```python
from build123d import *

# Parameters (mm, degrees)
F1_DEPTH = 7.62
F2_R     = 2.365375
F3_DEPTH = 25.4


with BuildPart() as f1:
    # F0 (on Front) → F1 (new body)
    with BuildSketch(Plane.XZ):
        Polygon((10.0597376004, 17.4239766347), (-10.0597376004, 17.4239766347), (-20.1194752008, 0), (-10.0597376004, -17.4239766347), (10.0597376004, -17.4239766347), (20.1194752008, 0), align=None)
        with BuildLine():
            add(Edge.make_bspline(
                [(-8.8631942381, -0.7304763376), (-8.451958628, -1.1782662241), (-8.451958628, -1.8910746148)],
                knots=[0, 0, 0, 1, 1, 1], degree=2))
            add(Edge.make_bspline(
                [(-8.451958628, -1.8910746148), (-8.451958628, -2.8095008106), (-9.1183126258, -3.3243068706)],
                knots=[0, 0, 0, 1, 1, 1], degree=2))
            add(Edge.make_bspline(
                [(-9.1183126258, -3.3243068706), (-9.7846666235, -3.8391129306), (-10.9269877626, -3.8391129306)],
                knots=[0, 0, 0, 1, 1, 1], degree=2))
            add(Edge.make_bspline(
                [(-10.9269877626, -3.8391129306), (-12.1637407824, -3.8391129306), (-12.8308563276, -3.5192630116)],
                knots=[0, 0, 0, 1, 1, 1], degree=2))
            Line((-12.8308563276, -3.5192630116), (-12.8308563276, -2.7394384474))
            add(Edge.make_bspline(
                [(-12.8308563276, -2.7394384474), (-12.4013435793, -2.9191636399), (-11.8971991833, -3.0242571847)],
                knots=[0, 0, 0, 1, 1, 1], degree=2))
            add(Edge.make_bspline(
                [(-11.8971991833, -3.0242571847), (-11.3930547873, -3.1293507295), (-10.8980489604, -3.1293507295)],
                knots=[0, 0, 0, 1, 1, 1], degree=2))
            add(Edge.make_bspline(
                [(-10.8980489604, -3.1293507295), (-10.0892855939, -3.1293507295), (-9.6795730788, -2.8224471168)],
                knots=[0, 0, 0, 1, 1, 1], degree=2))
            add(Edge.make_bspline(
                [(-9.6795730788, -2.8224471168), (-9.2698605636, -2.5155435042), (-9.2698605636, -1.9672293574)],
                knots=[0, 0, 0, 1, 1, 1], degree=2))
            add(Edge.make_bspline(
                [(-9.2698605636, -1.9672293574), (-9.2698605636, -1.6062558775), (-9.4153161219, -1.3755070074)],
                knots=[0, 0, 0, 1, 1, 1], degree=2))
            add(Edge.make_bspline(
                [(-9.4153161219, -1.3755070074), (-9.5607716803, -1.1447581373), (-9.9011833797, -0.9490404489)],
                knots=[0, 0, 0, 1, 1, 1], degree=2))
            add(Edge.make_bspline(
                [(-9.9011833797, -0.9490404489), (-10.2415950792, -0.7533227604), (-10.9361263317, -0.5065813943)],
                knots=[0, 0, 0, 1, 1, 1], degree=2))
            add(Edge.make_bspline(
                [(-10.9361263317, -0.5065813943), (-11.9063377524, -0.1593157681), (-12.3229041944, 0.3166513732)],
                knots=[0, 0, 0, 1, 1, 1], degree=2))
            add(Edge.make_bspline(
                [(-12.3229041944, 0.3166513732), (-12.7394706365, 0.7926185144), (-12.7394706365, 1.558735225)],
                knots=[0, 0, 0, 1, 1, 1], degree=2))
            add(Edge.make_bspline(
                [(-12.7394706365, 1.558735225), (-12.7394706365, 2.3629293069), (-12.1355635276, 2.8388964481)],
                knots=[0, 0, 0, 1, 1, 1], degree=2))
            add(Edge.make_bspline(
                [(-12.1355635276, 2.8388964481), (-11.5316564188, 3.3148635894), (-10.5355523856, 3.3148635894)],
                knots=[0, 0, 0, 1, 1, 1], degree=2))
            add(Edge.make_bspline(
                [(-10.5355523856, 3.3148635894), (-9.4983247914, 3.3148635894), (-8.627114536, 2.9340898764)],
                knots=[0, 0, 0, 1, 1, 1], degree=2))
            Line((-8.627114536, 2.9340898764), (-8.8799482814, 2.2304200547))
            add(Edge.make_bspline(
                [(-8.8799482814, 2.2304200547), (-9.7420199677, 2.5913935347), (-10.5553526187, 2.5913935347)],
                knots=[0, 0, 0, 1, 1, 1], degree=2))
            add(Edge.make_bspline(
                [(-10.5553526187, 2.5913935347), (-11.1980986462, 2.5913935347), (-11.5598336736, 2.3157133664)],
                knots=[0, 0, 0, 1, 1, 1], degree=2))
            add(Edge.make_bspline(
                [(-11.5598336736, 2.3157133664), (-11.9215687009, 2.0400331982), (-11.9215687009, 1.5495966559)],
                knots=[0, 0, 0, 1, 1, 1], degree=2))
            add(Edge.make_bspline(
                [(-11.9215687009, 1.5495966559), (-11.9215687009, 1.1886231759), (-11.7882979014, 0.9571127584)],
                knots=[0, 0, 0, 1, 1, 1], degree=2))
            add(Edge.make_bspline(
                [(-11.7882979014, 0.9571127584), (-11.6550271018, 0.7256023409), (-11.3382233726, 0.5329308422)],
                knots=[0, 0, 0, 1, 1, 1], degree=2))
            add(Edge.make_bspline(
                [(-11.3382233726, 0.5329308422), (-11.0214196434, 0.3402593434), (-10.3695350467, 0.107225831)],
                knots=[0, 0, 0, 1, 1, 1], degree=2))
            add(Edge.make_bspline(
                [(-10.3695350467, 0.107225831), (-9.2744298481, -0.2826864511), (-8.8631942381, -0.7304763376)],
                knots=[0, 0, 0, 1, 1, 1], degree=2))
        make_face(mode=Mode.SUBTRACT)
        Polygon((-1.8158343578, -3.7431579549), (-2.6535365264, -3.7431579549), (-3.5201774972, -1.5301011349), (-6.3089641712, -1.5301011349), (-7.1649434781, -3.7431579549), (-7.9843685085, -3.7431579549), (-5.2336592057, 3.2448012262), (-4.5528358069, 3.2448012262), align=None, mode=Mode.SUBTRACT)
        with BuildLine():
            Line((1.4024650645, -0.8492777361), (-0.0505674243, -0.8492777361))
            Line((-0.0505674243, -0.8492777361), (-0.0505674243, -3.7431579549))
            Line((-0.0505674243, -3.7431579549), (-0.8593307907, -3.7431579549))
            Line((-0.8593307907, -3.7431579549), (-0.8593307907, 3.215862424))
            Line((-0.8593307907, 3.215862424), (1.0491070589, 3.215862424))
            add(Edge.make_bspline(
                [(1.0491070589, 3.215862424), (2.3300298294, 3.215862424), (2.9415524125, 2.7254258816)],
                knots=[0, 0, 0, 1, 1, 1], degree=2))
            add(Edge.make_bspline(
                [(2.9415524125, 2.7254258816), (3.5530749956, 2.2349893393), (3.5530749956, 1.24954697)],
                knots=[0, 0, 0, 1, 1, 1], degree=2))
            add(Edge.make_bspline(
                [(3.5530749956, 1.24954697), (3.5530749956, -0.1303769659), (2.1533508266, -0.6162442237)],
                knots=[0, 0, 0, 1, 1, 1], degree=2))
            Line((2.1533508266, -0.6162442237), (4.0435115379, -3.7431579549))
            Line((4.0435115379, -3.7431579549), (3.0870079709, -3.7431579549))
            Line((3.0870079709, -3.7431579549), (1.4024650645, -0.8492777361))
        make_face(mode=Mode.SUBTRACT)
        Polygon((10.3780630275, -3.7431579549), (9.5403608589, -3.7431579549), (8.6737198881, -1.5301011349), (5.884933214, -1.5301011349), (5.0289539072, -3.7431579549), (4.2095288768, -3.7431579549), (6.9602381795, 3.2448012262), (7.6410615784, 3.2448012262), align=None, mode=Mode.SUBTRACT)
    extrude(amount=F1_DEPTH)

    # F2 (on face) → F3 (cut)
    with BuildSketch(Plane.XZ.offset(7.62)):
        with Locations((6.8676967915, 11.7051630221)):
            Circle(F2_R)
    extrude(amount=-F3_DEPTH, mode=Mode.SUBTRACT)


solid = f1.part
```
CAD build for the part. Positions are in the model's coordinates, mm. A direction names the side the tool comes from. Round coordinates to 2 decimals unless told otherwise and drop trailing zeros. Loops run counter-clockwise (first coordinate to the right, second up) from the corner with the lowest first, then second, coordinate; pieces in that order, holes last. Notation, with made-up numbers: (43, 7) - (80, 7) arc R18 ccw to (80, 22) - close; hole circle Ø7 at (-27.75, 85). An arc over 180 degrees is marked (long way). Return JSON: item names as keys, results as strings. Group by question number.
Q1. Drill centre lines: line 1 along Z through (x, y) = (1, -4.75); line 2 along X through (y, z) = (-2.5, 1); line 3 along Z through (x, y) = (-5, -1). Where is each one in solid material? Low to high. Write a range as [from, to].
Q2. Two-plate mould, pull along Z, no slides. Class faces 3 (the face through (-15.16, -3.76, -8.59)), 4 (the face through (-0.051, -4, -2)), 5 (the face through (0, -4, 17.424)): +Z half, -Z half, draft (parallel to the pull), parting line (faces both ways), or undercut.
Q3. Flat gauge pins, fed straight in: pin 1 Ø2.5 at (y, z) = (-5, -3) entering from -X; pin 2 Ø5.5 at (x, z) = (6.87, 11.71) entering from +Y. Where does each tip first touch, or does it go through?
Q4. Band-saw the part on C-C on z = -14. Give the cut face in (x, y), plus the area to 3 significant figures.
Q5. Band-saw the part on A-A on z = -2. Give the number of separate pieces and of enclosed holes in the cut face, plus the area to 3 significant figures.
Q6. Band-saw the part on D-D on x = -13.5. Give the cut face in (y, z).
Q7. Tool access for faces 1 (the face through (0, -4, -17.424)), 2 (the face through (-6.73, -3.76, -2.62)): list every direction of +Z, -Z, +X, -X, +Y, -Y with a clear straight run to the whole face (end or side of a thin tool).
Solutions:
{
 "1": {"line 1": "z = [-17.42, -0.85], [3.22, 17.42]", "line 2": "x = [-19.54, -12.67], [-11.81, -6.12], [-3.67, -0.86], [3.54, 6.08], [8.52, 19.54]", "line 3": "z = [-17.42, -1.53], [3.24, 17.42]"},
 "2": {"face 3": "-Z half", "face 4": "undercut", "face 5": "+Z half"},
 "3": {"pin 1": "stops at x = -19.11", "pin 2": "stops at y = 0"},
 "4": {"outline": "(-12.04, -7.62) - (12.04, -7.62) - (12.04, 0) - (-12.04, 0) - close", "area": "183 mm^2"},
 "5": {"separate pieces": "8", "enclosed holes": "0", "area": "245 mm^2"},
 "6": {"outline": "(-7.62, -11.47) - (0, -11.47) - (0, 11.47) - (-7.62, 11.47) - close"},
 "7": {"face 1": "-Z, +X, -X, +Y, -Y", "face 2": "+Y, -Y"}
}
